from build123d import *

# Parameters (mm, degrees)
ESQUISSE1_W             = 80
ESQUISSE1_H             = 80
BOSS_EXTRU_1_DEPTH      = 80
ESQUISSE1_4_R           = 20
ESQUISSE1_4_R_2         = 1.5
ENL_V_MAT_EXTRU_1_DEPTH = 3


with BuildPart() as part:
    # Esquisse1 → Boss.-Extru.1 (new body)
    with BuildSketch(Plane.XY):
        Rectangle(ESQUISSE1_W, ESQUISSE1_H)
    extrude(amount=BOSS_EXTRU_1_DEPTH)

    # Esquisse1<4> → Enlèv. mat.-Extru.1 (cut)
    with BuildSketch(Plane.XY):
        Circle(ESQUISSE1_4_R)
        with Locations((15, 0)):
            Circle(ESQUISSE1_4_R_2, mode=Mode.SUBTRACT)
    extrude(amount=ENL_V_MAT_EXTRU_1_DEPTH, mode=Mode.SUBTRACT)


solid = part.part
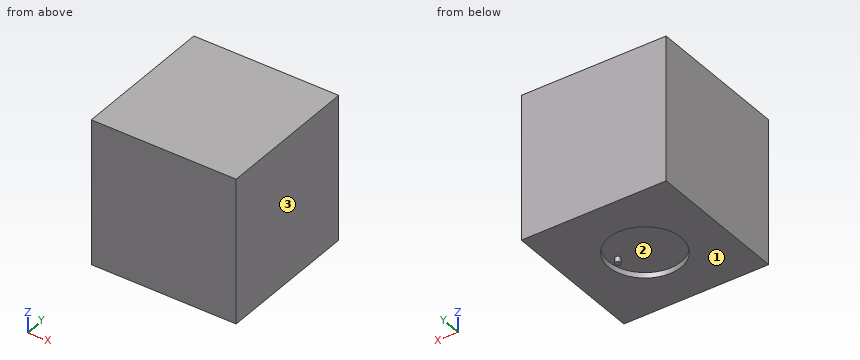
Input: part model. Units: mm. Frame: model coordinates. Face numbers are marked on the shaded views. Round coordinates to 2 decimals unless told otherwise and drop trailing zeros. Order: outer loops, then holes, each group sorted by start corner. A loop starts at its lowest first (then second) coordinate and runs counter-clockwise, first axis right, second up. Notation, with made-up numbers: (-25, 49.5) - (11, 49.5) arc R25 ccw to (11, 84.5) - close; hole circle Ø7 at (41.5, -39.5). An arc over 180 degrees is marked (long way). Answer as a JSON object with one key per item and string values. Group by question number.
(1) Cut plane C-C (y = -8). Return loops of the section in (x, z).
(2) Cut plane B-B (y = 0). Return loops of the section in (x, z).
(3) Pin query (flat end, axial travel): P1, Ø12, axis at x = 7.5, y = 10, coming from the -Z side. Return the tip coordinate at first contact, or that it passes through.
(4) Draft query along X for the marked faces 1, 2 and 3. Return one class per face: released by +X, released by -X, zero draft, split by the parting line, or undercut.
(5) Material intervals for probe 1 along Y at (x, z) = (0, 2.1); probe 2 along Z at (x, y) = (-15, -12), sorted ascending. Write a range as from..to.
(6) Cut plane A-A (x = 0). Return loops of the section in (y, z), then the cut area to 3 significant figures.
Here are the results:
{
 "1": {"outline": "(-40, 0) - (-18.33, 0) - (-18.33, 3) - (18.33, 3) - (18.33, 0) - (40, 0) - (40, 80) - (-40, 80) - close"},
 "2": {"outline": "(-40, 0) - (-20, 0) - (-20, 3) - (13.5, 3) - (13.5, 0) - (16.5, 0) - (16.5, 3) - (20, 3) - (20, 0) - (40, 0) - (40, 80) - (-40, 80) - close"},
 "3": {"P1": "stops at z = 3"},
 "4": {"face 1": "zero draft", "face 2": "undercut", "face 3": "released by +X"},
 "5": {"probe 1": "y = -40..-20, 20..40", "probe 2": "z = 3..80"},
 "6": {"outline": "(-40, 0) - (-20, 0) - (-20, 3) - (20, 3) - (20, 0) - (40, 0) - (40, 80) - (-40, 80) - close", "area": "6,280 mm^2"}
}
